The figure shows three views and two pictorial views of one solid part (mm, origin at its lowest corner). Answer the questions. A direction names the side the tool comes from. Give positions to 0.01 mm unless a question says otherwise; leave off trailing zeros. Order: outer loops, then holes, each group sorted by start corner. A loop starts at its lowest first (then second) coordinate and runs counter-clockwise, first axis right, second up. Notation, with made-up numbers: (50, -31.5) - (102, -31.5) arc R19 ccw to (102, -8.5) - close; hole circle Ø9 at (11, -32.5). An arc over 180 degrees is marked (long way). Answer as CSV lines item,"result". Start each with the question number.
1. Flat-ended cylindrical pins translate along their axes: pin 1 (1 mm diameter, centred on y = 9.5, z = 3.5, fed in from -X); pin 2 (1.5 mm diameter, centred on y = 17, z = 2.5, fed in from +X); pin 3 (11 mm diameter, centred on x = 26, y = 11.5, fed in from +Z). Find the tip coordinate at first contact, or state that the pin passes through.
2. Consider line 1 along Y through (x, z) = (21.5, 0.6); line 2 along X through (y, z) = (8.5, 3.5); line 3 along Y through (x, z) = (4, 1). Determine where each line is inside the solid, lowest interval first. Write a range as [from, to].
3. Section B-B on z = 0.75 is taken. Give the vertices of the cut face in (x, y), and give its area (3 significant figures).
4. Section D-D on z = 6 is taken. Give the vertices of the cut face in (x, y).
5. Section C-C on x = 29 is taken. Give the vertices of the cut face in (y, z).
6. Section A-A on x = 4 is taken. Give the vertices of the cut face in (y, z).
7. Which of the six approach directions +Z, -Z, +X, -X, +Y, -Y give full straight-line access (tool end or side, diameter ignored) to the marked faces 1 and 2?
8. Determine the mould class of the marked faces 3, 4, 5 and 6 for opening direction Y: +Y half, -Y half, draft (parallel to the pull), parting line (faces both ways), or undercut.
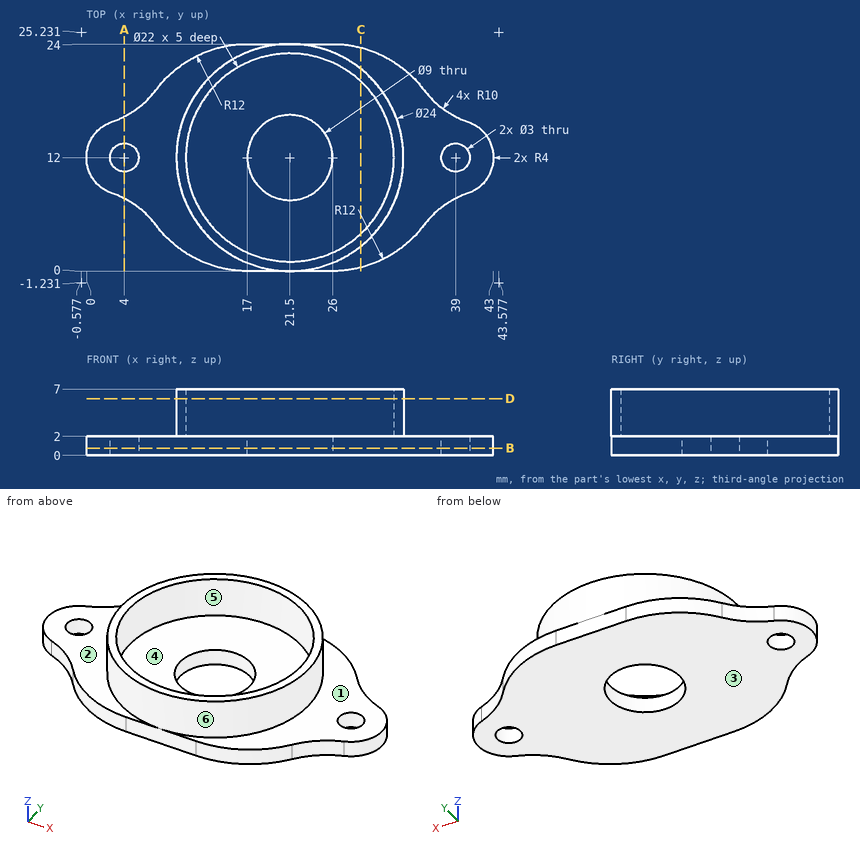
Checks:
1,pin 1,"stops at x = 9.67"
1,pin 2,"stops at x = 38.81"
1,pin 3,"stops at z = 2"
2,line 1,"y = [0, 7.5], [16.5, 24]"
2,line 2,"x = [10.02, 11.07], [31.93, 32.98]"
2,line 3,"y = [7.66, 10.5], [13.5, 16.34]"
3,outline,"(2.69, 8.22) arc R10 cw to (7.41, 4.78) arc R12 ccw to (17, 0) - (26, 0) arc R12 ccw to (35.59, 4.78) arc R10 cw to (40.31, 8.22) arc R4 ccw to (40.31, 15.78) arc R10 cw to (35.59, 19.22) arc R12 ccw to (26, 24) - (17, 24) arc R12 ccw to (7.41, 19.22) arc R10 cw to (2.69, 15.78) arc R4 ccw to start; hole circle Ø3 at (4, 12); hole circle Ø9 at (21.5, 12); hole circle Ø3 at (39, 12)"
3,area,"670 mm²"
4,outline,"circle Ø24 at (21.5, 12); hole circle Ø22 at (21.5, 12)"
5,outline,"(0.38, 0) - (23.62, 0) - (23.62, 2) - (21.37, 2) - (21.37, 7) - (20.05, 7) - (20.05, 2) - (3.95, 2) - (3.95, 7) - (2.63, 7) - (2.63, 2) - (0.38, 2) - close"
6,outline,"(7.66, 0) - (10.5, 0) - (10.5, 2) - (7.66, 2) - close; (13.5, 0) - (16.34, 0) - (16.34, 2) - (13.5, 2) - close"
7,face 1,"+Z, +X"
7,face 2,"+Z, -X"
8,face 3,"draft"
8,face 4,"undercut"
8,face 5,"undercut"
8,face 6,"parting line"
